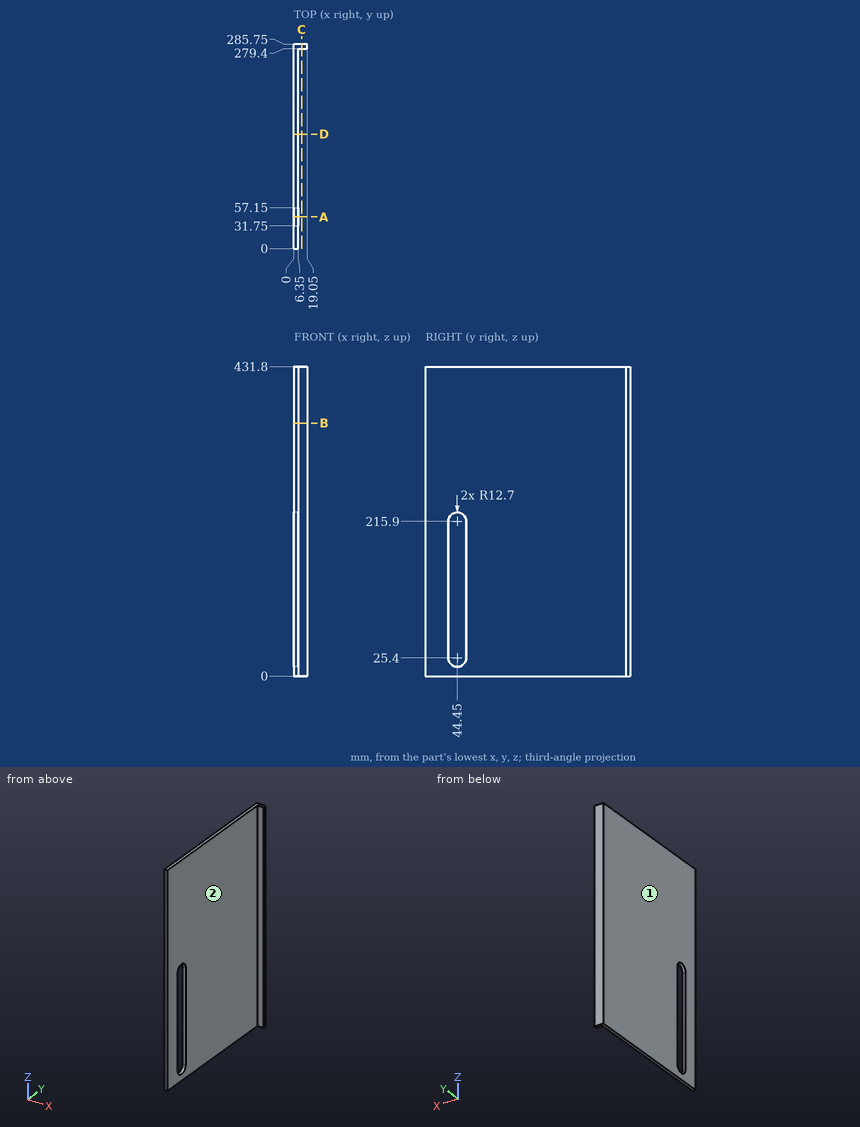
Source: three-view drawing plus pictorial views. Frame: mm from the lowest corner of the part. A direction names the side the tool comes from. Round coordinates to 2 decimals unless told otherwise and drop trailing zeros. Loops run counter-clockwise (first coordinate to the right, second up) from the corner with the lowest first, then second, coordinate; pieces in that order, holes last. Notation, with made-up numbers: (86, 57.25) -> (98, 57.25) arc R16 cw to (98, 66.25) -> close; hole circle Ø3 at (-35, 3). An arc over 180 degrees is marked (long way). Use one line per item in the form item = value.
Item 1: Cut plane D-D on y = 160. Output: boundary loops of the cut face in (x, z).
Evaluation:
outline = (0, 0) -> (6.35, 0) -> (6.35, 431.8) -> (0, 431.8) -> close
Item 2: Cut plane C-C on x = 10.75. Output: boundary loops of the cut face in (y, z), then the cut area to 3 significant figures.
Evaluation:
outline = (279.4, 0) -> (285.75, 0) -> (285.75, 431.8) -> (279.4, 431.8) -> close
area = 2,740 mm2
Item 3: Cut plane A-A on y = 44.45. Output: boundary loops of the cut face in (x, z), then the cut area to 3 significant figures.
Evaluation:
outline = (0, 0) -> (6.35, 0) -> (6.35, 12.7) -> (0, 12.7) -> close; (0, 228.6) -> (6.35, 228.6) -> (6.35, 431.8) -> (0, 431.8) -> close
area = 1,370 mm2
Item 4: Material intervals for probe 1 along Y at (x, z) = (3.25, 33); probe 2 along X at (y, z) = (221, 380); probe 3 along Y at (x, z) = (18, 387.5), sorted ascending.
Evaluation:
probe_1 = 0 to 31.75, 57.15 to 285.75
probe_2 = 0 to 6.35
probe_3 = 279.4 to 285.75
Item 5: Cut plane B-B on z = 353. Output: boundary loops of the cut face in (x, y), then the cut area to 3 significant figures.
Evaluation:
outline = (0, 0) -> (6.35, 0) -> (6.35, 279.4) -> (19.05, 279.4) -> (19.05, 285.75) -> (0, 285.75) -> close
area = 1,900 mm2
Item 6: Access query for the marked faces 1 and 2. Directions: +Z, -Z, +X, -X, +Y, -Y. A direction counts if a zero-diameter tool reaches every point of the face in a straight line with its end or side. Return the directions, or none.
Evaluation:
face_1 = +Z, -Z, -X, +Y, -Y
face_2 = +Z, -Z, +X, -Y
Item 7: Contact query for a flat-ended pin moving along its axis: pin 1 Ø4 at (x, z) = (9.5, 228) entering from -Y. Output: stop coordinate, or through.
Evaluation:
pin_1 = 279.4
